For this review, take the finished solid that the model builds, in its own axes (mm). A direction names the side the tool comes from. Coordinates: 2 decimals unless noted, no trailing zeros. Write each loop counter-clockwise with the first axis right and the second up, starting at its lowest first coordinate (ties: lowest second). Pieces come first, ordered by that corner, then holes. Notation, with made-up numbers: (59, 65.5) - (79, 65.5) arc R31 cw to (79, 102.5) - close; hole circle Ø4 at (7.25, -35). An arc over 180 degrees is marked (long way). Write each question's results on one line, items separated by ' | '.
from build123d import *

# Parameters (mm, degrees)
RESSALTO_EXTRUS_O1_DEPTH = 4
CORTE_EXTRUS_O3_DEPTH    = 116.464280191
ESBO_O4_W                = 4
ESBO_O4_H                = 20
RESSALTO_EXTRUS_O2_DEPTH = 4


with BuildPart() as part:
    # Esboço1 → Ressalto-extrusão1 (new body)
    with BuildSketch(Plane.XY):
        Polygon((-50, -100), (-37, -100), (-37, -104), (-13, -104), (-13, -100), (13, -100), (13, -104), (37, -104), (37, -100), (50, -100), (50, 100), (-50, 100), align=None)
    extrude(amount=RESSALTO_EXTRUS_O1_DEPTH)

    # Esboço2 → Corte-extrusão3 (cut, through all)
    with BuildSketch(Plane.XY.offset(4)):
        Polygon((0, 20), (0, 0), (50, 0), (50, 100), (0, 100), (0, 80), (4, 80), (4, 60), (0, 60), (0, 40), (4, 40), (4, 20), align=None)
        Polygon((0, -80), (0, -100), (13, -100), (13, -104), (37, -104), (37, -100), (50, -100), (50, 0), (0, 0), (0, -20), (4, -20), (4, -40), (0, -40), (0, -60), (4, -60), (4, -80), align=None)
    extrude(amount=-CORTE_EXTRUS_O3_DEPTH, mode=Mode.SUBTRACT)

    # Esboço4 → Ressalto-extrusão2 (add)
    with BuildSketch(Plane.XY.offset(4)):
        with Locations((-52, 70)):
            Rectangle(ESBO_O4_W, ESBO_O4_H)
        with Locations((-52, 30)):
            Rectangle(ESBO_O4_W, ESBO_O4_H)
        with Locations((-52, -70)):
            Rectangle(ESBO_O4_W, ESBO_O4_H)
        with Locations((-52, -30)):
            Rectangle(ESBO_O4_W, ESBO_O4_H)
    extrude(amount=-RESSALTO_EXTRUS_O2_DEPTH)


solid = part.part
Q1. Wall thickness on line 1 along Y through (x, z) = (1, 1.3); line 2 along X through (y, z) = (-14, 2.8); line 3 along Y through (x, z) = (-1, 0.95): over which ranges is each line inside the solid? List them lowest first. Write a range as from..to.
Results found:
line 1: -80..-60, -40..-20, 20..40, 60..80 | line 2: -50..0 | line 3: -100..100
Q2. Take a section at B-B on x = -40. State the section outline as (y, z) points, plus the area to 3 significant figures.
Results found:
outline: (-100, 0) - (100, 0) - (100, 4) - (-100, 4) - close | area: 800 mm2
Q3. For pin 1 (1.2 mm diameter, centred on y = -46.5, z = 2, fed in from +X); pin 2 (6 mm diameter, centred on x = -20.5, y = -46, fed in from -Z); pin 3 (2 mm diameter, centred on y = -52.5, z = 3.5, fed in from -X), all flat-tipped, find the tip position at first contact; note any pin that passes through.
Results found:
pin 1: x = 0 | pin 2: z = 0 | pin 3: x = -50
Q4. Take a section at A-A on y = 83. State the section outline as (x, z) points, plus the area to 3 significant figures.
Results found:
outline: (-50, 0) - (0, 0) - (0, 4) - (-50, 4) - close | area: 200 mm2
Q5. Mouldability with a two-part tool opening along Y and no side actions: class faces 6 (the face through (4, 70, 2)), 7 (the face through (-52, -60, 2)), 8 (the face through (-44, -100, 2)) as pulls with the +Y half, pulls with the -Y half, needs draft (parallel to the pull), parting line crosses it, or undercut.
Results found:
face 6: needs draft | face 7: undercut | face 8: pulls with the -Y half
Q6. For faces 1 (the face through (0, 50, 2)), 2 (the face through (2, 80, 2)), 3 (the face through (-52, 40, 2)), 4 (the face through (4, -30, 2)), 5 (the face through (-13, -102, 2)), list the 3-axis set-ups (+Z, -Z, +X, -X, +Y, -Y) from which the entire face can be reached by the end or side of a thin tool; tool diameter is ignored.
Results found:
face 1: +Z, -Z, +X | face 2: +Z, -Z, +X, +Y | face 3: +Z, -Z, -X | face 4: +Z, -Z, +X, +Y, -Y | face 5: +Z, -Z, +X, -Y
